The listing builds one solid part. Answer for the finished solid, in the listing's coordinates (mm). Face numbers are marked on the shaded views. Give positions to 0.01 mm unless a question says otherwise; leave off trailing zeros. Use a Markdown table: item, result. Add a question column.
1) Straight lines are drawn through the part: line 1 (X direction, y = 2.75, z = 18); line 2 (Z direction, x = 40.5, y = 9.75); line 3 (X direction, y = -10.5, z = -8.5). For each, find the intervals that lie inside material, in ascending order.
2) The mould has two halves that part along Z. Classify the marked faces 1, 2, 3 and 4: released by +Z, released by -Z, zero draft, split by the parting line, or undercut.
3) Flat-ended cylindrical pins translate along their axes: pin 1 (12 mm diameter, centred on y = 1, z = -9, fed in from -X); pin 2 (7 mm diameter, centred on y = -3, z = 2, fed in from +X); pin 3 (1 mm diameter, centred on y = -1, z = 5, fed in from -X). Find the tip coordinate at first contact, or state that the pin passes through.
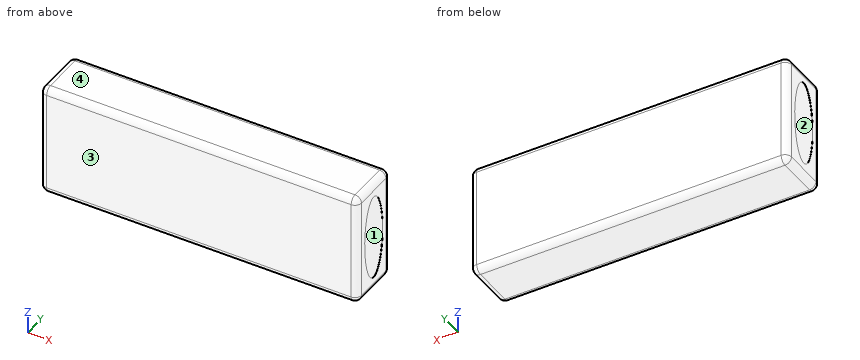
from build123d import *

# Parameters (mm, degrees)
RESSALTO_EXTRUS_O1_DEPTH      = 12.5
RESSALTO_EXTRUS_O1_DEPTH_BACK = 12.5
ESBO_O1_W                     = 147
ESBO_O1_H                     = 52
FILETE1_R                     = 3
FILETE2_R                     = 3
ESBO_O2_RX                    = 20
ESBO_O2_RY                    = 7
CORTE_EXTRUS_O1_DEPTH         = 0.1
ESBO_O3_RX                    = 20
ESBO_O3_RY                    = 7
CORTE_EXTRUS_O2_DEPTH         = 0.1


with BuildPart() as part:
    # Esboço1 → Ressalto-extrusão1 (new, two sides: drawn at the far end of the back side and taken through both)
    with BuildSketch(Plane(origin=(0, 0, 0), x_dir=(1, 0, 0), z_dir=(0, 1, 0)).offset(-RESSALTO_EXTRUS_O1_DEPTH_BACK)):
        Rectangle(ESBO_O1_W, ESBO_O1_H)
    extrude(amount=RESSALTO_EXTRUS_O1_DEPTH + RESSALTO_EXTRUS_O1_DEPTH_BACK)

    # Filete1
    filete1_edges = [part.edges().sort_by_distance(p)[0] for p in [
        (0, 12.5, -26),
        (0, -12.5, 26),
        (0, 12.5, 26),
        (0, -12.5, -26),
    ]]
    fillet(filete1_edges, radius=FILETE1_R)

    # Filete2
    filete2_edges = [part.edges().sort_by_distance(p)[0] for p in [
        (73.5, 0, 26),
        (-73.5, 0, 26),
        (73.5, 0, -26),
        (73.5, 12.5, 0),
        (73.5, -12.5, 0),
        (73.5, 11.621320344, 25.121320344),
        (73.5, 11.621320344, -25.121320344),
        (73.5, -11.621320344, -25.121320344),
        (73.5, -11.621320344, 25.121320344),
        (-73.5, -12.5, 0),
        (-73.5, 12.5, 0),
        (-73.5, 0, -26),
        (-73.5, 11.621320344, 25.121320344),
        (-73.5, 11.621320344, -25.121320344),
        (-73.5, -11.621320344, -25.121320344),
        (-73.5, -11.621320344, 25.121320344),
    ]]
    fillet(filete2_edges, radius=FILETE2_R)

    # Esboço2 → Corte-extrusão1 (cut)
    with BuildSketch(Plane(origin=(73.5, 0, 0), x_dir=(0, 0, -1), z_dir=(1, 0, 0))):
        with Locations((0, 0)):
            Ellipse(ESBO_O2_RX, ESBO_O2_RY)
    extrude(amount=-CORTE_EXTRUS_O1_DEPTH, mode=Mode.SUBTRACT)

    # Esboço3 → Corte-extrusão2 (cut)
    with BuildSketch(Plane.ZY.offset(73.5)):
        with Locations(Location((0, 0), (0, 0, 180))):
            Ellipse(ESBO_O3_RX, ESBO_O3_RY)
    extrude(amount=-CORTE_EXTRUS_O2_DEPTH, mode=Mode.SUBTRACT)


solid = part.part
The answers:
| question | item | result |
|---|---|---|
| 1 | line 1 | -73.4 to 73.4 |
| 1 | line 2 | -25.99 to 25.99 |
| 1 | line 3 | -73.33 to 73.33 |
| 2 | face 1 | undercut |
| 2 | face 2 | undercut |
| 2 | face 3 | zero draft |
| 2 | face 4 | released by +Z |
| 3 | pin 1 | x = -73.5 |
| 3 | pin 2 | x = 73.4 |
| 3 | pin 3 | x = -73.4 |
